Geometry check sheet. Reference: the model listing, model coordinates, mm. Coordinates: 2 decimals unless noted, no trailing zeros. Write each loop counter-clockwise with the first axis right and the second up, starting at its lowest first coordinate (ties: lowest second). Pieces come first, ordered by that corner, then holes. Notation, with made-up numbers: M 33,-14 L 55,-14 A16 ccw 55,4 Z; hole C 71.25,76 d5. An arc over 180 degrees is marked long. Put each result on its own line as item: value. Start each with the question number.
1) Cross-section at D-D on y = 45. Record the cut outline in (x, z).
2) Mould release check, pull along X, two halves, no side actions. Record for faces 1 (the flat face through (180, 33, -2)), 2 (the flat face through (89, 67, -2)), 3 (the cylindrical face through (9.733, 59.033, -1.232)): released by +X, released by -X, zero draft, split by the parting line, or undercut.
3) Cross-section at B-B on z = -1.1. Count the separate pieces of the cut face and the enclosed holes in it, plus the area to 3 significant figures.
4) Scan lines: line 1 along Y through (x, z) = (105.75, -1.55); line 2 along Y through (x, z) = (104, -4.75); line 3 along X through (y, z) = (15, -2.85). Record each from-to range of solid material in increasing order.
5) Cross-section at A-A on x = 105.75. Record the cut outline in (y, z), plus the area to 4 significant figures.
6) Gauge pin test, flat end, axial feed: pin 1 (3.5 mm diameter, centred on x = 130, y = 53.5, fed in from -Z). Record the tip position at first contact, or that the pin passes through.
7) Cross-section at C-C on x = 58. Record the cut outline in (y, z).
from build123d import *

# Parameters (mm, degrees)
F0_W     = 180
F0_H     = 67
F0_R     = 2.05
F0_R_2   = 3.05
F0_R_3   = 8
F1_DEPTH = 5
F2_SIZE  = 3.5
F3_SIZE  = 2.5


with BuildPart() as f1:
    # F0 (on Top) → F1 (new body)
    with BuildSketch(Plane.XY):
        with Locations((90, 33.5)):
            Rectangle(F0_W, F0_H)
        with Locations((10, 10)):
            Circle(F0_R, mode=Mode.SUBTRACT)
        with Locations((105.75, 10)):
            Circle(F0_R, mode=Mode.SUBTRACT)
        with Locations((130, 13.5)):
            Circle(F0_R_2, mode=Mode.SUBTRACT)
        with Locations((170, 13.5)):
            Circle(F0_R_2, mode=Mode.SUBTRACT)
        with Locations((58, 41.5)):
            Circle(F0_R_3, mode=Mode.SUBTRACT)
        with Locations((10, 57)):
            Circle(F0_R, mode=Mode.SUBTRACT)
        with Locations((105.75, 57)):
            Circle(F0_R, mode=Mode.SUBTRACT)
        with Locations((130, 53.5)):
            Circle(F0_R_2, mode=Mode.SUBTRACT)
        with Locations((170, 53.5)):
            Circle(F0_R_2, mode=Mode.SUBTRACT)
    extrude(amount=-F1_DEPTH)

    # F2
    f2_edges = [f1.edges().sort_by_distance(p)[0] for p in [
        (126.95, 53.5, 0),
        (166.95, 53.5, 0),
        (166.95, 13.5, 0),
        (126.95, 13.5, 0),
    ]]
    chamfer(f2_edges, length=F2_SIZE)

    # F3
    f3_edges = [f1.edges().sort_by_distance(p)[0] for p in [
        (103.7, 57, -5),
        (103.7, 10, -5),
        (7.95, 10, -5),
        (7.95, 57, -5),
    ]]
    chamfer(f3_edges, length=F3_SIZE)


solid = f1.part
Answer key:
1. outline: M 0,-5 L 50.81,-5 L 50.81,0 L 0,0 Z; M 65.19,-5 L 180,-5 L 180,0 L 65.19,0 Z
2. face 1: released by +X
2. face 2: zero draft
2. face 3: undercut
3. separate pieces: 1
3. enclosed holes: 9
3. area: 11,400 mm²
4. line 1: y = 0 to 7.95, 12.05 to 54.95, 59.05 to 67
4. line 2: y = 0 to 6.07, 13.93 to 53.07, 60.93 to 67
4. line 3: x = 0 to 126.62, 133.38 to 166.62, 173.38 to 180
5. outline: M 0,-5 L 5.45,-5 L 7.95,-2.5 L 7.95,0 L 0,0 Z; M 12.05,-2.5 L 14.55,-5 L 52.45,-5 L 54.95,-2.5 L 54.95,0 L 12.05,0 Z; M 59.05,-2.5 L 61.55,-5 L 67,-5 L 67,0 L 59.05,0 Z
5. area: 281.5 mm²
6. pin 1: passes through
7. outline: M 0,-5 L 33.5,-5 L 33.5,0 L 0,0 Z; M 49.5,-5 L 67,-5 L 67,0 L 49.5,0 Z
